```python
from build123d import *

# Parameters (mm, degrees)
SKETCH2_W          = 3.2
SKETCH2_H          = 6.1
CUT_EXTRUDE1_DEPTH = 2
CUT_EXTRUDE2_REACH = 17.838
SKETCH3_R          = 1


with BuildPart() as part:
    # Sketch1 → Revolve1 (revolve)
    with BuildSketch(Plane.XY):
        with BuildLine():
            Line((0, 8), (0, 7.5))
            ThreePointArc((0, 7.5), (-5.303300859, 5.303300859), (-7.5, 0))
            Line((-7.5, 0), (-8, 0))
            ThreePointArc((-8, 0), (-5.656854249, 5.656854249), (0, 8))
        make_face()
    revolve(axis=Axis((-8, 0, 0), (1, 0, 0)))

    # Sketch2 → Cut-Extrude1 (cut)
    with BuildSketch(Plane.XY.offset(8)):
        Rectangle(SKETCH2_W, SKETCH2_H)
    extrude(amount=-CUT_EXTRUDE1_DEPTH, mode=Mode.SUBTRACT)

    # Sketch3 → Cut-Extrude2 (cut, up to next)
    with BuildSketch(Plane.XY.offset(-8), mode=Mode.PRIVATE) as cut_extrude2_sk1:
        Circle(SKETCH3_R)
    cut_extrude2_tool1 = extrude(cut_extrude2_sk1.sketch, amount=CUT_EXTRUDE2_REACH, mode=Mode.PRIVATE) & part.part
    add(cut_extrude2_tool1.solids().sort_by_distance((0, 0, -8))[0], mode=Mode.SUBTRACT)


solid = part.part
```
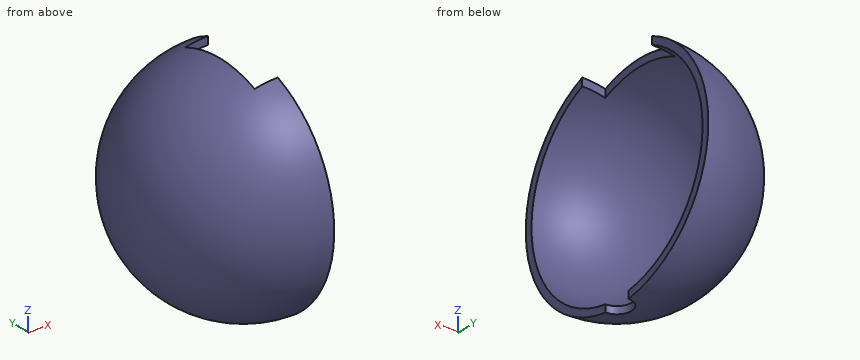
The model under review builds one solid part; all positions refer to its coordinate system, in mm. Coordinates: 2 decimals unless noted, no trailing zeros. Order: outer loops, then holes, each group sorted by start corner. A loop starts at its lowest first (then second) coordinate and runs counter-clockwise, first axis right, second up. Notation, with made-up numbers: (31.5, 22) -> (49.5, 22) arc R22 ccw to (49.5, 32) -> close; hole circle Ø11 at (-1, -19.75). An arc over 180 degrees is marked (long way). Answer in a Markdown table with one row per item. Add a question column.
Item 1: To check wall thickness, follow probe 1 along Y at (x, z) = (-1.75, -0.5); probe 2 along Y at (x, z) = (-3.5, 3.5); probe 3 along Z at (x, y) = (-6.5, 1). State the ranges of each line that lie inside material, in increasing order.
Item 2: We need section D-D on z = -6.25. Write out the cut boundary in (x, y).
Item 3: We need section B-B on y = 0. Write out the cut boundary in (x, z).
Item 4: We need section C-C on x = -4.75. Write out the cut boundary in (y, z).
Item 5: We need section A-A on x = -0.75. Write out the cut boundary in (y, z), plus the area to 3 significant figures.
Item 6: Clearance check with flat-ended pins moving along their axes: pin 1 (8 mm diameter, centred on y = -2.5, z = 1, fed in from +X); pin 2 (3 mm diameter, centred on x = -1.5, z = -2, fed in from -Y); pin 3 (4 mm diameter, centred on x = -3.5, z = 0.5, fed in from +Y). State where each tip first meets the part, or that it passes through.
Final values:
| question | item | result |
|---|---|---|
| 1 | probe 1 | y = -7.79 to -7.28, 7.28 to 7.79 |
| 1 | probe 2 | y = -6.28 to -5.63, 5.63 to 6.28 |
| 1 | probe 3 | z = -4.56 to -3.61, 3.61 to 4.56 |
| 2 | outline | (0, -4.99) -> (0, -4.15) arc R4.15 cw to (0, 4.15) -> (0, 4.99) arc R4.99 ccw to start |
| 3 | outline | (-1.6, 7.33) -> (-1.6, 7.84) arc R8 ccw to (-1, -7.94) -> (-1, -7.43) arc R7.5 cw to start |
| 4 | outline | circle Ø12.87 at (0, 0); hole circle Ø11.61 at (0, 0) |
| 5 | outline | (-3.05, 6.81) -> (-3.05, 7.36) arc R7.96 ccw to (-0.66, -7.94) -> (-0.66, -7.43) arc R7.46 cw to start; (0.66, -7.94) arc R7.96 ccw to (3.05, 7.36) -> (3.05, 6.81) arc R7.46 cw to (0.66, -7.43) -> close |
| 5 | area | 20.5 mm2 |
| 6 | pin 1 | stops at x = -3.39 |
| 6 | pin 2 | stops at y = -7.94 |
| 6 | pin 3 | stops at y = 7.85 |
